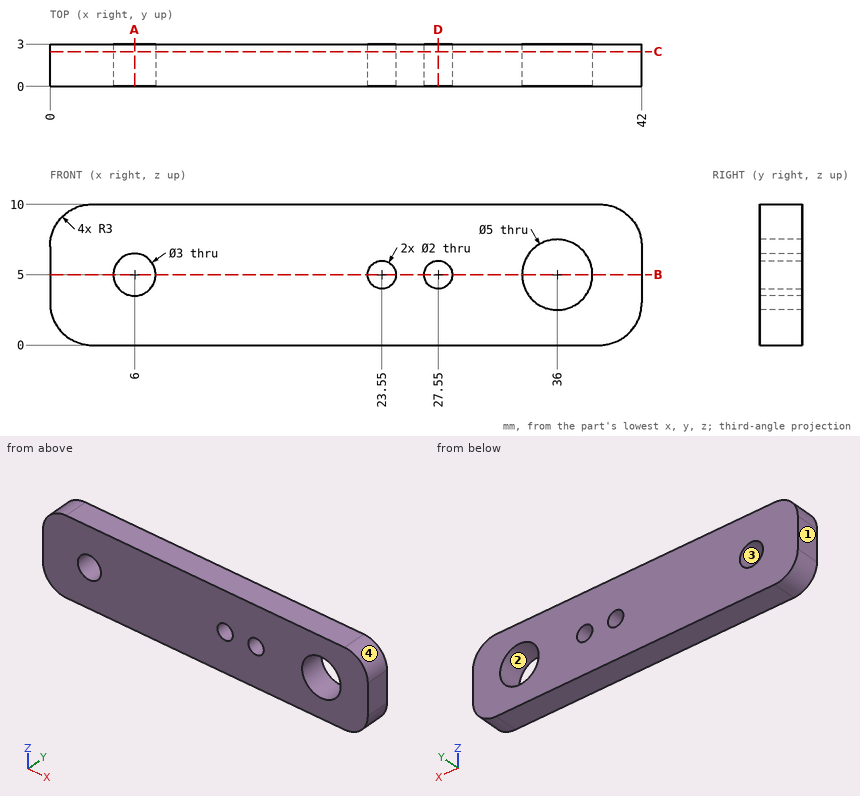
Could you check a few things on this drawing? It's one solid part, dimensions in mm from its lowest x, y, z. Round coordinates to 2 decimals unless told otherwise and drop trailing zeros. Write each loop counter-clockwise with the first axis right and the second up, starting at its lowest first coordinate (ties: lowest second). Pieces come first, ordered by that corner, then holes.
Q1. If we mould it in two halves opening along Z, with no side actions, what happens to the marked faces 1, 2, 3 and 4? For each: +Z half, -Z half, draft (parallel to the pull), parting line (faces both ways), or undercut.
Q2. Will these pins go through, and if not, where does the flat tip stop? P1, Ø1.8, axis at x = 27.55, z = 5, coming from the -Y side; P2, Ø5, axis at x = 6, z = 5, coming from the -Y side.
Q3. If we section it at C-C on y = 2.45: Write out the boundary of the cut face in (x, z).
Q4. If we section it at D-D on x = 27.55: Write out the boundary of the cut face in (y, z).
Q5. If we section it at A-A on x = 6: Write out the boundary of the cut face in (y, z), plus the area to 3 significant figures.
Q6. Please list where these lines run through material, in increasing order: probe 1 along Z at (x, y) = (27.55, 1.3); probe 2 along Z at (x, y) = (6, 2); probe 3 along X at (y, z) = (1.25, 5.5).
Q7. If we section it at B-B on z = 5: Write out the boundary of the cut face in (x, y).
Answer below:
1. face 1: draft
1. face 2: undercut
1. face 3: undercut
1. face 4: +Z half
2. P1: passes through
2. P2: stops at y = 0
3. outline: (0, 3) arc R3 ccw to (3, 0) - (39, 0) arc R3 ccw to (42, 3) - (42, 7) arc R3 ccw to (39, 10) - (3, 10) arc R3 ccw to (0, 7) - close; hole circle Ø3 at (6, 5); hole circle Ø2 at (23.55, 5); hole circle Ø2 at (27.55, 5); hole circle Ø5 at (36, 5)
4. outline: (0, 0) - (3, 0) - (3, 4) - (0, 4) - close; (0, 6) - (3, 6) - (3, 10) - (0, 10) - close
5. outline: (0, 0) - (3, 0) - (3, 3.5) - (0, 3.5) - close; (0, 6.5) - (3, 6.5) - (3, 10) - (0, 10) - close
5. area: 21.0 mm2
6. probe 1: z = 0 to 4, 6 to 10
6. probe 2: z = 0 to 3.5, 6.5 to 10
6. probe 3: x = 0 to 4.59, 7.41 to 22.68, 24.42 to 26.68, 28.42 to 33.55, 38.45 to 42
7. outline: (0, 0) - (4.5, 0) - (4.5, 3) - (0, 3) - close; (7.5, 0) - (22.55, 0) - (22.55, 3) - (7.5, 3) - close; (24.55, 0) - (26.55, 0) - (26.55, 3) - (24.55, 3) - close; (28.55, 0) - (33.5, 0) - (33.5, 3) - (28.55, 3) - close; (38.5, 0) - (42, 0) - (42, 3) - (38.5, 3) - close
